Verification items for the finished model (mm, model axes). A direction names the side the tool comes from. Give positions to 0.01 mm unless a question says otherwise; leave off trailing zeros. Write each loop counter-clockwise with the first axis right and the second up, starting at its lowest first coordinate (ties: lowest second). Pieces come first, ordered by that corner, then holes. Notation, with made-up numbers: (56.25, -23) - (85.25, -23) arc R22 cw to (85.25, -7) - close; hole circle Ø3 at (22.5, 60). An arc over 180 degrees is marked (long way). Answer as a JSON object with one key per item and string values. Group by question number.
Item 1: Sectioned sample at D-D, the plane x = -55.5. Record the boundary of the cut face in (y, z).
Item 2: Sectioned sample at B-B, the plane y = 42. Record the boundary of the cut face in (x, z), and give its area (3 significant figures).
Item 3: Draft check along X on faces 1 (the face through (-22.406, 67.719, -145.07)), 2 (the face through (-29.508, 45.304, -143.451)), 3 (the face through (-60, 36, -60)), 4 (the face through (-35, 40, -55)). Enter one of: +X half, -X half, draft (parallel to the pull), parting line (faces both ways), or undercut.
Item 4: Scan lines: line 1 along Y through (x, z) = (-40, -56); line 2 along Z through (x, y) = (-26, 18); line 3 along Y through (x, z) = (-40, -61). Record each from-to range of solid material in increasing order. Write a range as [from, to].
Item 5: Go/stop test with flat-tipped pins: pin 1 (11 mm diameter, centred on y = 25.5, z = -60.5, fed in from +X); pin 2 (5 mm diameter, centred on x = -40, y = 42, fed in from -Z); pin 3 (3 mm diameter, centred on y = 28.5, z = -147, fed in from -X); pin 4 (8 mm diameter, centred on x = -55.5, z = -74.5, fed in from +Y). Record where each tip stops, or that it passes through.
Item 6: Tool access check on faces 5 (the face through (-20, 36, -60)), 6 (the face through (-31, 33, -140)), 7 (the face through (-60, 36, -145)), 8 (the face through (-40, 37, -58)). Record the directions out of +Z, -Z, +X, -X, +Y, -Y that give a thin tool (end or side, any length) a straight path to the whole face; none if there is none.
Item 7: Sectioned sample at C-C, the plane z = -19.5. Record the boundary of the cut face in (x, y), and give its area (3 significant figures).
Item 8: Sectioned sample at A-A, the plane x = -40. Record the boundary of the cut face in (y, z).
Autodesk Inventor part; units mm, degrees
ref_plane "YZ Plane" through (0, 0, 0) normal (1, 0, 0) x (0, 1, 0)
ref_plane "XZ Plane" through (0, 0, 0) normal (0, 1, 0) x (-1, 0, 0)
ref_plane "XY Plane" through (0, 0, 0) normal (0, 0, 1) x (1, 0, 0)
sketch "Boceto1" plane through (0, 0, 0) normal (0, 1, 0) x (-1, 0, 0)
  line L0 (0, 0) -> (80, 0)
  line L1 (80, 0) -> (80, -150)
  line L2 (80, -150) -> (0, -150)
  line L3 (0, -150) -> (0, 0)
  line L4 (80, -150) -> (0, -150)
  line L5 (0, -150) -> (0, -140)
  line L6 (0, -140) -> (80, -140)
  line L7 (80, -140) -> (80, -150)
  line L8 (80, -65) -> (0, -65)
  line L9 (0, -65) -> (0, -55)
  line L10 (0, -55) -> (80, -55)
  line L11 (80, -55) -> (80, -65)
  line L12 (80, -25) -> (0, -25)
  line L13 (0, -25) -> (0, -15)
  line L14 (0, -15) -> (80, -15)
  line L15 (80, -15) -> (80, -25)
  point P0 (0, -65)
  point P1 (0, -15)
  point P2 (0, -25)
  point P3 (0, -55)
  point P4 (80, -55)
  dimension "d0" = 80
  dimension "d1" = 150
  dimension "d4" = 80
  dimension "d5" = 10
  dimension "d6" = 80
  dimension "d7" = 10
  dimension "d8" = 80
  dimension "d9" = 10
  dimension "d17" = 75
  dimension "d19" = 30
extrude "Extrusión1" add sketch "Boceto1" along normal blind 10 contours L0 L1 L14 L3 | L12 L1 L10 L3 | L8 L1 L6 L3
extrude "Extrusión2" add sketch "Boceto1" along normal blind 70 contours L14 L1 L12 L3 | L10 L1 L8 L3 | L6 L1 L2 L3
sketch "Boceto3" plane through (0, 0, -150) normal (0, 0, -1) x (-1, 0, 0)
  circle A0 centre (40, 42) radius 4
  line L0 (0, 0) -> (0, 70)
  line L1 (0, 70) -> (80, 70)
  line L2 (80, 10) -> (0, 10)
  circle A1 centre (40, 42) radius 11
  dimension "d12" = 8
  dimension "d13" = 40
  dimension "d18" = 32
  dimension "d54" = 22
extrude "Extrusión3" cut sketch "Boceto3" against normal blind 10 contours A0
sketch "Boceto4" plane through (-80, 10, -15) normal (0, 0, 1) x (1, 0, 0)
  circle A0 centre (40, 32) radius 4
  circle A1 centre (40, 32) radius 4
  circle A2 centre (40, 32) radius 12.5
  circle A3 centre (24.5, 47.4996) radius 1.5
  circle A4 centre (55.5, 47.4996) radius 1.5
  circle A5 centre (24.5009, 16.4996) radius 1.5
  circle A6 centre (55.4991, 16.4996) radius 1.5
  point P0 (80, -10)
  dimension "d20" = 8
  dimension "d21" = 25
  dimension "d26" = 3
  dimension "d27" = 21.92
  dimension "d28" = 3
  dimension "d29" = 21.92
  dimension "d30" = 3
  dimension "d31" = 3
  dimension "d32" = 21.92
  dimension "d33" = 21.92
  dimension "d47" = 0
  dimension "d48" = 31
  dimension "d51" = 0
  dimension "d53" = 31
extrude "Extrusión4" cut sketch "Boceto4" against normal blind 10 contours A0
extrude "Extrusión6" cut sketch "Boceto4" against normal blind 8 contours A2
sketch "Boceto5" plane through (0, 10, -65) normal (0, 0, -1) x (-1, 0, 0)
  circle A0 centre (40, 32) radius 4
  circle A1 centre (40, 32) radius 4
  point P0 (0, -10)
  dimension "d44" = 8
extrude "Extrusión7" cut sketch "Boceto5" against normal blind 10
sketch "Boceto6" plane through (-80, 10, -140) normal (0, 0, 1) x (1, 0, 0)
  circle A0 centre (40, 32) radius 4
  circle A1 centre (40, 32) radius 11
  point P0 (80, -10)
  dimension "d55" = 22
extrude "Extrusión8" cut sketch "Boceto6" against normal blind 7
sketch "Boceto7" plane through (-80, 10, -15) normal (0, 0, 1) x (1, 0, 0)
  line L0 (0, -10) -> (0, 60)
  line L1 (0, 0) -> (80, 0)
  line L2 (0, 60) -> (20, 60)
  line L3 (20, 60) -> (20, 0)
  line L4 (20, 0) -> (0, 0)
  line L5 (0, 0) -> (0, 60)
  line L6 (80, 60) -> (60, 60)
  line L7 (60, 60) -> (60, 0)
  line L8 (60, 0) -> (80, 0)
  line L9 (80, 0) -> (80, 60)
  point P0 (80, -10)
  dimension "d58" = 20
  dimension "d59" = 20
extrude "Extrusión9" cut sketch "Boceto7" against normal blind 150
fillet "Empalme1" radius 8 1 edges at (-20, 70, -20)
fillet "Empalme2" radius 8 1 edges at (-60, 70, -20)
fillet "Empalme3" radius 8 1 edges at (-60, 70, -60)
fillet "Empalme4" radius 8 1 edges at (-20, 70, -60)
fillet "Empalme5" radius 8 1 edges at (-60, 70, -145)
fillet "Empalme6" radius 8 1 edges at (-20, 70, -145)
sketch "Boceto8" plane through (-20, 10, -65) normal (0, 0, -1) x (-1, 0, 0)
  circle A0 centre (20, 32) radius 11
  circle A1 centre (20, 32) radius 11
  point P0 (-20, -10)
  dimension "d68" = 22
extrude "Extrusión10" cut sketch "Boceto8" against normal blind 7
sketch "Boceto9" plane through (-80, 0, 0) normal (0, 0, 1) x (1, 0, 0)
  line L0 (0, 0) -> (80, 0)
  line L1 (0, 10) -> (10, 10)
  line L2 (10, 10) -> (10, 0)
  line L3 (10, 0) -> (0, 0)
  line L4 (0, 0) -> (0, 10)
  line L5 (0, 10) -> (80, 10)
  line L6 (80, 10) -> (70, 10)
  line L7 (70, 10) -> (70, 0)
  line L8 (70, 0) -> (80, 0)
  line L9 (80, 0) -> (80, 10)
  dimension "d71" = 10
  dimension "d72" = 10
extrude "Extrusión11" cut sketch "Boceto9" against normal blind 150 contours L4 L1 L2 L0 | L7 L5 L9 L0
sketch "Boceto10" plane through (-60, 10, -15) normal (0, 0, 1) x (1, 0, 0)
  line L0 (0, 52) -> (0, 0)
  line L1 (0, 0) -> (40, 0)
  line L2 (40, 0) -> (40, 60)
  line L3 (40, 60) -> (0, 60)
  line L4 (0, 60) -> (0, 0)
  point P0 (60, -10)
  dimension "d75" = 40
  dimension "d76" = 60
extrude "Extrusión12" cut sketch "Boceto10" against normal blind 10
properties part number "SOPORTE - INFERIOR"
Geometry check:
{
 "1": {"outline": "(0, -150) - (69.19, -150) - (69.19, -140) - (10, -140) - (10, -65) - (69.19, -65) - (69.19, -55) - (10, -55) - (10, 0) - (0, 0) - close"},
 "2": {"outline": "(-60, -150) - (-44, -150) - (-44, -147) - (-51, -147) - (-51, -140) - (-60, -140) - close; (-60, -65) - (-51, -65) - (-51, -58) - (-44, -58) - (-44, -55) - (-60, -55) - close; (-36, -150) - (-20, -150) - (-20, -140) - (-29, -140) - (-29, -147) - (-36, -147) - close; (-36, -58) - (-29, -58) - (-29, -65) - (-20, -65) - (-20, -55) - (-36, -55) - close", "area": "444 mm^2"},
 "3": {"face 1": "+X half", "face 2": "undercut", "face 3": "-X half", "face 4": "draft"},
 "4": {"line 1": "[0, 38], [46, 70]", "line 2": "[-150, -140], [-65, -55]", "line 3": "[0, 31], [53, 70]"},
 "5": {"pin 1": "x = -20", "pin 2": "through", "pin 3": "x = -60", "pin 4": "y = 10"},
 "6": {"face 5": "+Z, -Z, +X, +Y", "face 6": "+X, -X, +Y", "face 7": "+Z, -Z, -X, +Y", "face 8": "none"},
 "7": {"outline": "(-70, 0) - (-10, 0) - (-10, 10) - (-70, 10) - close", "area": "600 mm^2"},
 "8": {"outline": "(0, -150) - (38, -150) - (38, -147) - (31, -147) - (31, -140) - (10, -140) - (10, -65) - (31, -65) - (31, -58) - (38, -58) - (38, -55) - (10, -55) - (10, 0) - (0, 0) - close; (46, -150) - (70, -150) - (70, -140) - (53, -140) - (53, -147) - (46, -147) - close; (46, -58) - (53, -58) - (53, -65) - (70, -65) - (70, -55) - (46, -55) - close"}
}
